Build history of the part. All positions in model axes, mm. A direction names the side the tool comes from. Round coordinates to 2 decimals unless told otherwise and drop trailing zeros. Order: outer loops, then holes, each group sorted by start corner. A loop starts at its lowest first (then second) coordinate and runs counter-clockwise, first axis right, second up. Notation, with made-up numbers: (-5.5, -27.75) -> (17.5, -27.75) arc R32 cw to (17.5, 8.25) -> close; hole circle Ø2 at (6.25, 1). An arc over 180 degrees is marked (long way). Answer as a JSON object with one key per item and string values.
from build123d import *

# Parameters (mm, degrees)
F0_W     = 46.2
F0_H     = 46.2
F1_DEPTH = 166
F0_W_2   = 60
F0_H_2   = 60
F2_DEPTH = 4
F3_R     = 4
F4_R     = 2
F7_DEPTH = 80


with BuildPart() as f1:
    # F0 (on Top) → F1 (new body)
    with BuildSketch(Plane.XY):
        Polygon((27.65, 17.65), (27.65, 27.65), (-27.65, 27.65), (-27.65, 17.65), (-28.05, 17.65), (-28.05, 7.65), (-27.65, 7.65), (-27.65, -7.65), (-28.05, -7.65), (-28.05, -17.65), (-27.65, -17.65), (-27.65, -27.65), (-17.65, -27.65), (-17.65, -27.95), (-7.65, -27.95), (-7.65, -27.65), (7.65, -27.65), (7.65, -27.95), (17.65, -27.95), (17.65, -27.65), (27.65, -27.65), (27.65, -17.65), (28.05, -17.65), (28.05, -7.65), (27.65, -7.65), (27.65, 7.65), (28.05, 7.65), (28.05, 17.65), align=None)
        Rectangle(F0_W, F0_H, mode=Mode.SUBTRACT)
    extrude(amount=F1_DEPTH)

    # F0 (on Top) → F2 (join)
    with BuildSketch(Plane.XY):
        Rectangle(F0_W_2, F0_H_2)
        Polygon((-27.65, 27.65), (27.65, 27.65), (27.65, 17.65), (28.05, 17.65), (28.05, 7.65), (27.65, 7.65), (27.65, -7.65), (28.05, -7.65), (28.05, -17.65), (27.65, -17.65), (27.65, -27.65), (17.65, -27.65), (17.65, -27.95), (7.65, -27.95), (7.65, -27.65), (-7.65, -27.65), (-7.65, -27.95), (-17.65, -27.95), (-17.65, -27.65), (-27.65, -27.65), (-27.65, -17.65), (-28.05, -17.65), (-28.05, -7.65), (-27.65, -7.65), (-27.65, 7.65), (-28.05, 7.65), (-28.05, 17.65), (-27.65, 17.65), align=None, mode=Mode.SUBTRACT)
        Polygon((27.65, 17.65), (27.65, 27.65), (-27.65, 27.65), (-27.65, 17.65), (-28.05, 17.65), (-28.05, 7.65), (-27.65, 7.65), (-27.65, -7.65), (-28.05, -7.65), (-28.05, -17.65), (-27.65, -17.65), (-27.65, -27.65), (-17.65, -27.65), (-17.65, -27.95), (-7.65, -27.95), (-7.65, -27.65), (7.65, -27.65), (7.65, -27.95), (17.65, -27.95), (17.65, -27.65), (27.65, -27.65), (27.65, -17.65), (28.05, -17.65), (28.05, -7.65), (27.65, -7.65), (27.65, 7.65), (28.05, 7.65), (28.05, 17.65), align=None)
        Rectangle(F0_W, F0_H, mode=Mode.SUBTRACT)
    extrude(amount=-F2_DEPTH)

    # F3
    f3_edges = [f1.edges().sort_by_distance(p)[0] for p in [
        (-27.65, 27.65, 83),
        (-27.65, -27.65, 83),
        (27.65, -27.65, 83),
        (27.65, 27.65, 83),
        (30, 30, -2),
        (30, -30, -2),
        (-30, 30, -2),
        (-30, -30, -2),
    ]]
    fillet(f3_edges, radius=F3_R)

    # F4
    f4_edges = [f1.edges().sort_by_distance(p)[0] for p in [
        (30, 0, -4),
    ]]
    fillet(f4_edges, radius=F4_R)

    # F6 (on offset) → F7 (cut)
    with BuildSketch(Plane.XZ.offset(27.65)):
        with BuildLine():
            Line((-5.630705, 127.75), (-7.370688, 122.394882))
            ThreePointArc((-7.370688, 122.394882), (0, 112.25), (7.370688, 122.394882))
            Line((7.370688, 122.394882), (5.630705, 127.75))
            Line((5.630705, 127.75), (-5.630705, 127.75))
        make_face()
    extrude(amount=-F7_DEPTH, mode=Mode.SUBTRACT)


solid = f1.part
1) Cut at C-C, the plane x = 0. Give the cut face in (y, z), plus the area to 3 significant figures.
Checked values:
{"outline": "(-30, -2) arc R2 ccw to (-28, -4) -> (-23.1, -4) -> (-23.1, 112.25) -> (-27.65, 112.25) -> (-27.65, 0) -> (-30, 0) -> close; (-27.65, 127.75) -> (-23.1, 127.75) -> (-23.1, 166) -> (-27.65, 166) -> close; (23.1, -4) -> (28, -4) arc R2 ccw to (30, -2) -> (30, 0) -> (27.65, 0) -> (27.65, 112.25) -> (23.1, 112.25) -> close; (23.1, 127.75) -> (27.65, 127.75) -> (27.65, 166) -> (23.1, 166) -> close", "area": "1,420 mm²"}
2) Probe L1, parallel to X at y = 4, z = 4; L2, parallel to Z at x = 0, y = -24; L3, parallel to X at y = -17, z = 81.5. List the from-to ranges inside material, lowest first. Write a range as from..to.
Checked values:
{"L1": "x = -27.65..-23.1, 23.1..27.65", "L2": "z = -4..112.25, 127.75..166", "L3": "x = -28.05..-23.1, 23.1..28.05"}
3) Which spindle directions (+Z, -Z, +X, -X, +Y, -Y) get a long thin tool onto all of the face, cutting with end or side? Do faces 1 (the face through (27.65, 0, 82)), 2 (the face through (-27.65, 0, 82)), 3 (the face through (-26.447, -26.509, 84.162)), 4 (the face through (-6.49, 25.34, 125.11)), 5 (the face through (-28.05, -13, 82)). Say none if no direction does.
Checked values:
{"face 1": "+Z, +X", "face 2": "+Z, -X", "face 3": "+Z, -X, -Y", "face 4": "+Y, -Y", "face 5": "+Z, -X, +Y, -Y"}
4) Cut at A-A, the plane y = 2.5. Give the cut face in (x, z), plus the area to 3 significant figures.
Checked values:
{"outline": "(-30, -2) arc R2 ccw to (-28, -4) -> (-23.1, -4) -> (-23.1, 166) -> (-27.65, 166) -> (-27.65, 0) -> (-30, 0) -> close; (23.1, -4) -> (28, -4) arc R2 ccw to (30, -2) -> (30, 0) -> (27.65, 0) -> (27.65, 166) -> (23.1, 166) -> close", "area": "1,560 mm²"}
5) Flat gauge pins, fed straight in: pin 1 Ø5 at (x, y) = (19, -9) entering from +Z; pin 2 Ø8 at (x, z) = (8.5, 120.5) entering from +Y; pin 3 Ø8 at (x, y) = (-8, 19.5) entering from -Z; pin 4 Ø3 at (x, z) = (21.5, 111) entering from -Y. Where does each tip first touch, or does it go through?
Checked values:
{"pin 1": "passes through", "pin 2": "stops at y = 27.65", "pin 3": "stops at z = -4", "pin 4": "stops at y = -27.65"}
6) Cut at B-B, the plane x = 14. Give the cut face in (y, z), plus the area to 3 significant figures.
Checked values:
{"outline": "(-30, -2) arc R2 ccw to (-28, -4) -> (-23.1, -4) -> (-23.1, 166) -> (-27.95, 166) -> (-27.95, 0) -> (-30, 0) -> close; (23.1, -4) -> (28, -4) arc R2 ccw to (30, -2) -> (30, 0) -> (27.65, 0) -> (27.65, 166) -> (23.1, 166) -> close", "area": "1,610 mm²"}
7) Pull direction Z, two halves, no side cores. Call faces 6 (the face through (-25, 0, -4)), 7 (the face through (0, -25, 127.75)), 8 (the face through (23.1, 0, 82)), 9 (the face through (-6.49, -25.41, 125.11)): pulls with the +Z half, pulls with the -Z half, needs draft (parallel to the pull), parting line crosses it, or undercut.
Checked values:
{"face 6": "pulls with the -Z half", "face 7": "undercut", "face 8": "needs draft", "face 9": "undercut"}
